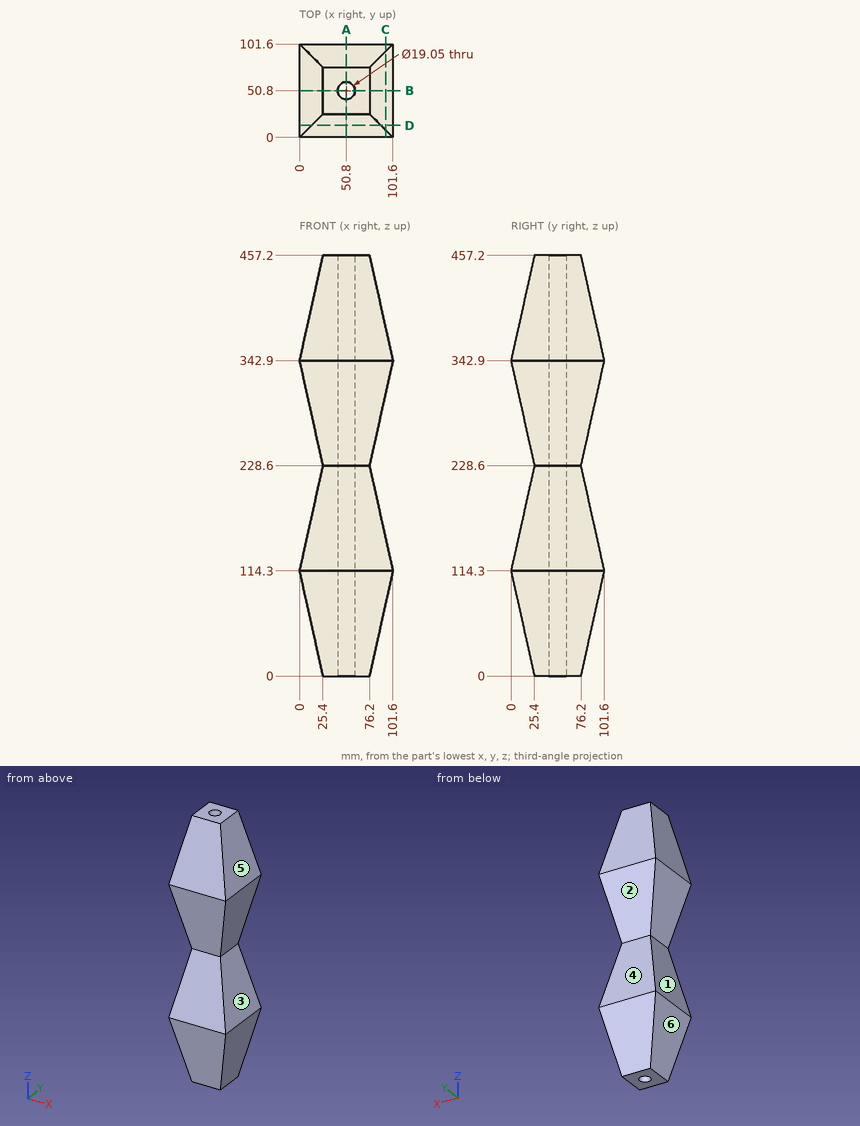
Design review of the part shown in the three views and the two pictorial views. Dimensions are in mm from the part's minimum x, y and z. A direction names the side the tool comes from. Round coordinates to 2 decimals unless told otherwise and drop trailing zeros. Write each loop counter-clockwise with the first axis right and the second up, starting at its lowest first coordinate (ties: lowest second). Pieces come first, ordered by that corner, then holes. Notation, with made-up numbers: (-24, -31.5) -> (31, -31.5) arc R20 cw to (31, -13.5) -> close; hole circle Ø2 at (7.25, -30). An arc over 180 degrees is marked (long way). Use one line per item in the form item = value.
1) Take a section at C-C, the plane x = 93.5. Write out the cut boundary in (y, z).
Found:
outline = (0, 114.3) -> (8.1, 77.85) -> (93.5, 77.85) -> (101.6, 114.3) -> (93.5, 150.75) -> (8.1, 150.75) -> close; (0, 342.9) -> (8.1, 306.45) -> (93.5, 306.45) -> (101.6, 342.9) -> (93.5, 379.35) -> (8.1, 379.35) -> close
2) To check wall thickness, follow L1, parallel to Y at x = 56, z = 261; L2, parallel to Y at x = 50, z = 136; L3, parallel to X at y = 50, z = 309. State the ranges of each line that lie inside material, in increasing order. Write a range as from..to.
Found:
L1 = 18.2..42.82, 58.78..83.4
L2 = 4.82..41.31, 60.29..96.78
L3 = 7.53..41.31, 60.29..94.07
3) Take a section at D-D, the plane y = 13. Write out the cut boundary in (x, z).
Found:
outline = (0, 114.3) -> (13, 55.8) -> (88.6, 55.8) -> (101.6, 114.3) -> (88.6, 172.8) -> (13, 172.8) -> close; (0, 342.9) -> (13, 284.4) -> (88.6, 284.4) -> (101.6, 342.9) -> (88.6, 401.4) -> (13, 401.4) -> close
4) Mouldability with a two-part tool opening along Z and no side actions: class the marked faces 4, 5 and 6 as +Z half, -Z half, draft (parallel to the pull), parting line (faces both ways), or undercut.
Found:
face_4 = undercut
face_5 = +Z half
face_6 = -Z half
5) Clearance check with flat-ended pins moving along their axes: pin 1 (1.5 mm diameter, centred on y = 88.5, z = 388.5, fed in from +X); pin 2 (12 mm diameter, centred on y = 75, z = 269, fed in from +X); pin 3 (1 mm diameter, centred on x = 31, z = 147, fed in from -Y). State where each tip first meets the part, or that it passes through.
Found:
pin_1 = 91.63
pin_2 = 86.51
pin_3 = 7.16
6) Tool access review of the marked faces 1, 2 and 3: name each direction out of +Z, -Z, +X, -X, +Y, -Y from which nothing blocks a thin tool from reaching the whole face with its end or side.
Found:
face_1 = -X, +Y, -Y
face_2 = +X, -X, +Y
face_3 = +X, +Y, -Y
7) Take a section at A-A, the plane x = 50.8. Write out the cut boundary in (y, z) (3 decimals), and give its area (3 significant figures).
Found:
outline = (0, 114.3) -> (25.4, 0) -> (41.275, 0) -> (41.275, 457.2) -> (25.4, 457.2) -> (0, 342.9) -> (25.4, 228.6) -> close; (60.325, 0) -> (76.2, 0) -> (101.6, 114.3) -> (76.2, 228.6) -> (101.6, 342.9) -> (76.2, 457.2) -> (60.325, 457.2) -> close
area = 26,100 mm2
